The listing builds one solid part. Answer for the finished solid, in the listing's coordinates (mm). Face numbers are marked on the shaded views. A direction names the side the tool comes from. Coordinates: 2 decimals unless noted, no trailing zeros. Order: outer loops, then holes, each group sorted by start corner. A loop starts at its lowest first (then second) coordinate and runs counter-clockwise, first axis right, second up. Notation, with made-up numbers: (2.25, 88.25) -> (33.25, 88.25) arc R11 cw to (33.25, 109.25) -> close; hole circle Ø8 at (78.25, 72). An arc over 180 degrees is marked (long way). Write item = value, one per line.
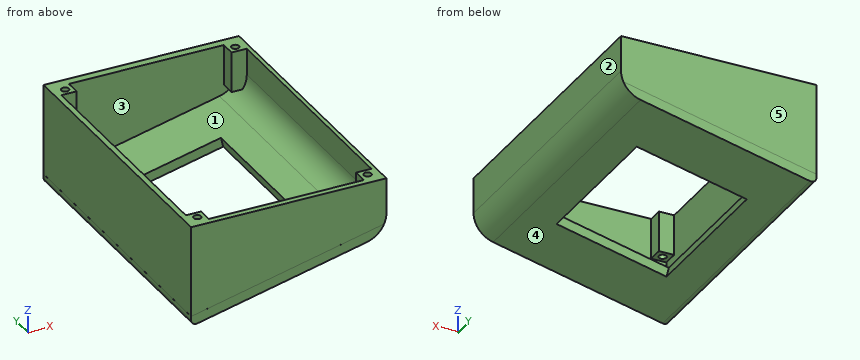
from build123d import *

# Parameters (mm, degrees)
RESSALTO_EXTRUS_O1_DEPTH   = 114
CORTE_EXTRUS_O1_DEPTH      = 59
RESSALTO_EXTRUS_O3_DEPTH   = 4
FILETE1_R                  = 10
FILETE2_R                  = 10
FILETE3_R                  = 10
FILETE4_R                  = 2
CORTE_EXTRUS_O2_DEPTH      = 19
CORTE_EXTRUS_O2_DEPTH_BACK = 10
F_3DSKETCH5_R              = 1.5
RESSALTO_EXTRUS_O6_DEPTH   = 16


with BuildPart() as part:
    # Esboço1 → Ressalto-extrusão1 (new body)
    with BuildSketch(Plane(origin=(0, 0, 0), x_dir=(1, 0, 0), z_dir=(0, 1, 0))):
        Polygon((113.296704203, 18.392857143), (190.296704203, 0.392857143), (190.296704203, -21.607142857), (113.296704203, -21.607142857), align=None)
    extrude(amount=RESSALTO_EXTRUS_O1_DEPTH)

    # 3DSketch1 → Corte-extrusão1 (cut)
    with BuildSketch(Plane(origin=(115.537266243, 110.682804253, 21.607142857), x_dir=(0.5597225204223067, -0.8286800951706879, 0), z_dir=(0, 0, -1))):
        Polygon((0, 0), (40.922432447, -60.586458429), (130.621864407, 0), (89.699431959, 60.586458429), align=None)
    extrude(amount=CORTE_EXTRUS_O1_DEPTH, mode=Mode.SUBTRACT)

    # 3DSketch3 → Ressalto-extrusão3 (add, along a direction that is not the sketch's normal)
    with BuildSketch(Plane(origin=(113.280710176, 114.017648872, -18.396596006), x_dir=(0.5549294721149596, -0.8217207699541985, 0.12972377270219831), z_dir=(-0.22762936703818706, 0, 0.9737478478855778))):
        Polygon((0, 0), (45.064591164, 64.978311237), (138.756352747, 0), (93.691761582, -64.978311237), align=None)
    extrude(amount=RESSALTO_EXTRUS_O3_DEPTH, dir=(0, 0, 1))

    # Filete1
    # the kernel refuses this fillet: 10 mm, written as the material it takes off along each edge
    with BuildSketch(Plane(origin=(190.296704203, -19.829841849, -0.392857143), x_dir=(-0.973747847885578, 0, -0.22762936703818593), z_dir=(0, 1, 0))) as filete1_piece_1:
        with BuildLine():
            CenterArc((FILETE1_R * 0.793193673946, FILETE1_R), FILETE1_R, 193.15754274, 76.84245726)
            Line((-FILETE1_R * 0.180554173939, FILETE1_R * 0.772370632962), (0, 0))
            Line((0, 0), (FILETE1_R * 0.793193673946, 0))
        make_face()
    extrude(amount=153.659683697, mode=Mode.SUBTRACT)

    # Filete2
    filete2_edges = [part.edges().sort_by_distance(p)[0] for p in [
        (188.649265411, 56.560934739, 3.222027295),
    ]]
    fillet(filete2_edges, radius=FILETE2_R)

    # Filete3
    filete3_edges = [part.edges().sort_by_distance(p)[0] for p in [
        (115.537266243, 56.560934739, -13.869089393),
    ]]
    fillet(filete3_edges, radius=FILETE3_R)

    # Filete4
    filete4_edges = [part.edges().sort_by_distance(p)[0] for p in [
        (113.280710176, 57.008160365, -18.396596006),
    ]]
    fillet(filete4_edges, radius=FILETE4_R)

    # 3DSketch4 → Corte-extrusão2 (cut, two sides: drawn at the far end of the back side and taken through both)
    with BuildSketch(Plane(origin=(170.820373008, 88.008160365, -4.945765734), x_dir=(-0.5677884026874886, -0.8124033121057346, -0.13272975647240007), z_dir=(0.22762936703818715, 0, -0.9737478478855778)).offset(-CORTE_EXTRUS_O2_DEPTH_BACK)):
        Polygon((0, 0), (25.94776869, 36.151947389), (76.316774041, 0), (50.369005351, -36.151947389), align=None)
    extrude(amount=CORTE_EXTRUS_O2_DEPTH + CORTE_EXTRUS_O2_DEPTH_BACK, mode=Mode.SUBTRACT)

    # 3DSketch5 → Ressalto-extrusão6 (add)
    # profile 1 of 4: a face of its own
    with BuildSketch(Plane(origin=(115.537266243, 110.682804253, 21.607142857), x_dir=(0.5597225204223067, -0.8286800951706879, 0), z_dir=(0, 0, -1))):
        Polygon((0, 0), (3.358335123, -4.972080571), (8.330415694, -1.613745448), (4.972080571, 3.358335123), align=None)
        with Locations(Location((4.165207847, -0.806872724, 0), (0, 0, 304.036610354))):
            Circle(F_3DSKETCH5_R, mode=Mode.SUBTRACT)
    # profile 2 of 4: a face of its own
    with BuildSketch(Plane(origin=(115.537266243, 110.682804253, 21.607142857), x_dir=(0.5597225204223067, -0.8286800951706879, 0), z_dir=(0, 0, -1))):
        Polygon((40.922432447, -60.586458429), (37.564097325, -55.614377858), (42.536177896, -52.256042735), (45.894513018, -57.228123306), align=None)
        with Locations(Location((41.729305172, -56.421250582, 0), (0, 0, 275.729153182))):
            Circle(F_3DSKETCH5_R, mode=Mode.SUBTRACT)
    # profile 3 of 4: a face of its own
    with BuildSketch(Plane(origin=(115.537266243, 110.682804253, 21.607142857), x_dir=(0.5597225204223067, -0.8286800951706879, 0), z_dir=(0, 0, -1))):
        Polygon((130.621864407, 0), (127.263529284, 4.972080571), (122.291448713, 1.613745448), (125.649783836, -3.358335123), align=None)
        with Locations(Location((126.45665656, 0.806872724, 0), (0, 0, 332.344067525))):
            Circle(F_3DSKETCH5_R, mode=Mode.SUBTRACT)
    # profile 4 of 4: a face of its own
    with BuildSketch(Plane(origin=(115.537266243, 110.682804253, 21.607142857), x_dir=(0.5597225204223067, -0.8286800951706879, 0), z_dir=(0, 0, -1))):
        Polygon((89.699431959, 60.586458429), (93.057767082, 55.614377858), (88.085686511, 52.256042735), (84.727351388, 57.228123306), align=None)
        with Locations(Location((88.892559235, 56.421250582, 0), (0, 0, 304.036610354))):
            Circle(F_3DSKETCH5_R, mode=Mode.SUBTRACT)
    extrude(amount=RESSALTO_EXTRUS_O6_DEPTH)


solid = part.part
Q1. The mould has two halves that part along Y. Classify the marked faces 3, 4 and 5: released by +Y, released by -Y, zero draft, split by the parting line, or undercut.
The answers:
face_3 = undercut
face_4 = zero draft
face_5 = released by +Y
Q2. Find the intervals of material crossed by line 1 along Y through (x, z) = (183.5, 12); line 2 along Y through (x, z) = (135, 11.5); line 3 along X through (y, z) = (95.5, 19), in increasing order.
The answers:
line_1 = 0 to 8.44, 104.68 to 114
line_2 = 0 to 2.44, 110.68 to 114
line_3 = 113.3 to 115.54, 188.65 to 190.3
Q3. Section C-C, the plane z = 14 is taken. Give the vertices of the cut face in (x, y).
The answers:
outline = (113.3, 0) -> (190.3, 0) -> (190.3, 114) -> (113.3, 114) -> close; hole (115.54, 8.44) -> (121.54, 8.44) -> (121.54, 2.44) -> (182.65, 2.44) -> (182.65, 8.44) -> (188.65, 8.44) -> (188.65, 104.68) -> (182.65, 104.68) -> (182.65, 110.68) -> (121.54, 110.68) -> (121.54, 104.68) -> (115.54, 104.68) -> close; hole circle Ø3 at (118.54, 5.44); hole circle Ø3 at (118.54, 107.68); hole circle Ø3 at (185.65, 5.44); hole circle Ø3 at (185.65, 107.68)
Q4. Each of these flat-tipped pins is pushed along its axis until it touches: pin 1 Ø5 at (x, y) = (176, 63) entering from -Z; pin 2 Ø1 at (x, z) = (162.5, 13) entering from +Y; pin 3 Ø3.5 at (x, y) = (185, 107) entering from -Z. Where does it stop, or does it pass through?
The answers:
pin_1 = -4.32
pin_2 = 114
pin_3 = -2.01
Q5. A tool of negligible diameter and unlimited length cuts with its end or side. For the marked faces 1 and 2, from which of +Z, -Z, +X, -X, +Y, -Y can it reach the whole face along a straight path? Write none if from no direction.
The answers:
face_1 = +Z
face_2 = +Z, -Z, +X, +Y, -Y
Q6. Section D-D, the plane x = 185.5 is taken. Give the number of separate pieces and of enclosed holes in the cut face, plus the area to 3 significant figures.
The answers:
separate_pieces = 3
enclosed_holes = 0
area = 754 mm2
